Check sheet for the modelled part. Datum: model origin and axes. Units: mm. A direction names the side the tool comes from. Round coordinates to 2 decimals unless told otherwise and drop trailing zeros. Write each loop counter-clockwise with the first axis right and the second up, starting at its lowest first coordinate (ties: lowest second). Pieces come first, ordered by that corner, then holes. Notation, with made-up numbers: M 23.5,-13 L 70.5,-13 A9 cw 70.5,-8 Z; hole C 25,-8 d4. An arc over 180 degrees is marked long. Answer in a Markdown table with one row per item.
```python
from build123d import *

# Parameters (mm, degrees)
SKETCH2_W           = 64
SKETCH2_H           = 22.3
SKETCH2_W_2         = 5
SKETCH2_H_2         = 5
BOSS_EXTRUDE1_DEPTH = 19
BOSS_EXTRUDE2_DEPTH = 8
SKETCH4_R           = 2.1
SKETCH4_W           = 5
SKETCH4_H           = 5.1
BOSS_EXTRUDE3_DEPTH = 2
SKETCH5_W           = 5
SKETCH5_H           = 5.1
SKETCH5_W_2         = 9
SKETCH5_H_2         = 22.3
BOSS_EXTRUDE4_DEPTH = 2.5


with BuildPart() as part:
    # Sketch2 → Boss-Extrude1 (new body)
    with BuildSketch(Plane.XY):
        Rectangle(SKETCH2_W, SKETCH2_H)
        with Locations((-34.5, 0)):
            Rectangle(SKETCH2_W_2, SKETCH2_H_2)
    extrude(amount=BOSS_EXTRUDE1_DEPTH)

    # Sketch3 → Boss-Extrude2 (add)
    with BuildSketch(Plane.XY):
        with BuildLine():
            ThreePointArc((-23, 1.825), (-23.707512696, 0), (-23, -1.825))
            Line((-23, -1.825), (-19, -1.825))
            ThreePointArc((-19, -1.825), (-18.475554477, -0.97867247), (-18.292487304, 0))
            ThreePointArc((-18.292487304, 0), (-18.475554477, 0.97867247), (-19, 1.825))
            Line((-19, 1.825), (-23, 1.825))
        make_face()
    extrude(amount=-BOSS_EXTRUDE2_DEPTH)

    # Sketch4 → Boss-Extrude3 (add)
    with BuildSketch(Plane(origin=(0, 0, 0), x_dir=(-1, 0, 0), z_dir=(0, 0, -1))):
        with Locations((10, 0)):
            Circle(SKETCH4_R)
        with Locations((-10, 0)):
            Rectangle(SKETCH4_W, SKETCH4_H)
    extrude(amount=BOSS_EXTRUDE3_DEPTH)

    # Sketch5 → Boss-Extrude4 (add)
    with BuildSketch(Plane.XY.offset(19)):
        with Locations((10, 0)):
            Rectangle(SKETCH5_W, SKETCH5_H)
        with Locations((26.5, 0)):
            Rectangle(SKETCH5_W_2, SKETCH5_H_2)
    extrude(amount=BOSS_EXTRUDE4_DEPTH)


solid = part.part
```
1. Section check B-B, the plane z = 5.5. Record the cut outline in (x, y), and give its area (3 significant figures).
Found:
| item | result |
|---|---|
| outline | M -37,-2.5 L -32,-2.5 L -32,-11.15 L 32,-11.15 L 32,11.15 L -32,11.15 L -32,2.5 L -37,2.5 Z |
| area | 1,450 mm2 |
2. Section check A-A, the plane x = 10.5. Record the cut outline in (y, z), and give its area (3 significant figures).
Found:
| item | result |
|---|---|
| outline | M -11.15,0 L -2.55,0 L -2.55,-2 L 2.55,-2 L 2.55,0 L 11.15,0 L 11.15,19 L 2.55,19 L 2.55,21.5 L -2.55,21.5 L -2.55,19 L -11.15,19 Z |
| area | 447 mm2 |
3. Section check D-D, the plane y = 0.75. Record the cut outline in (x, z), and give its area (3 significant figures).
Found:
| item | result |
|---|---|
| outline | M -37,0 L -23.6,0 L -23.6,-8 L -18.4,-8 L -18.4,0 L -11.96,0 L -11.96,-2 L -8.04,-2 L -8.04,0 L 7.5,0 L 7.5,-2 L 12.5,-2 L 12.5,0 L 32,0 L 32,19 L 31,19 L 31,21.5 L 22,21.5 L 22,19 L 12.5,19 L 12.5,21.5 L 7.5,21.5 L 7.5,19 L -37,19 Z |
| area | 1,410 mm2 |
4. Access from +Z, -Z, +X, -X, +Y, -Y to the whole of each face (thin tool, end or side, straight path). Record for faces 1 (the face through (7.5, 0, 20)), 2 (the face through (-21, -1.825, -4)), 3 (the face through (10, 2.55, -1)), 4 (the face through (-32, 7, 9)), 5 (the face through (-32, -7, 9)).
Found:
| item | result |
|---|---|
| face 1 | +Z, -X, +Y, -Y |
| face 2 | -Z, -X, -Y |
| face 3 | -Z, +X, -X, +Y |
| face 4 | +Z, -Z, -X, +Y |
| face 5 | +Z, -Z, -X, -Y |
5. Scan lines: L1, parallel to Z at x = -4.5, y = -5.5; L2, parallel to X at y = 3, z = 15; L3, parallel to Z at x = 27, y = 3.5. Record each from-to range of solid material in increasing order.
Found:
| item | result |
|---|---|
| L1 | z = 0 to 19 |
| L2 | x = -32 to 32 |
| L3 | z = 0 to 21.5 |
6. Draft check along X on faces 6 (the face through (-23.707, 0.028, -3.944)), 7 (the face through (-21, 1.825, -4)), 8 (the face through (12.5, 0, 20)). Enter one of: +X half, -X half, draft (parallel to the pull), parting line (faces both ways), or undercut.
Found:
| item | result |
|---|---|
| face 6 | -X half |
| face 7 | draft |
| face 8 | undercut |
7. Section check C-C, the plane y = -6.75. Record the cut outline in (x, z).
Found:
| item | result |
|---|---|
| outline | M -32,0 L 32,0 L 32,19 L 31,19 L 31,21.5 L 22,21.5 L 22,19 L -32,19 Z |
8. Go/stop test with flat-tipped pins: pin 1 (3.5 mm diameter, centred on x = -9.5, y = 1, fed in from -Z); pin 2 (4 mm diameter, centred on x = -35.5, z = 5.5, fed in from +Y); pin 3 (2.5 mm diameter, centred on y = -6, z = 7.5, fed in from -X). Record where each tip stops, or that it passes through.
Found:
| item | result |
|---|---|
| pin 1 | stops at z = -2 |
| pin 2 | stops at y = 2.5 |
| pin 3 | stops at x = -32 |
